Work out the finished part from the listing and answer in its coordinate system (mm). A direction names the side the tool comes from. Round coordinates to 2 decimals unless told otherwise and drop trailing zeros. Write each loop counter-clockwise with the first axis right and the second up, starting at its lowest first coordinate (ties: lowest second). Pieces come first, ordered by that corner, then holes.
1. A tool of negligible diameter and unlimited length cuts with its end or side. For faces 1 (the face through (2.98, -3.03, 3.05)), 2 (the face through (-2, -2, 1.5)), 3 (the face through (-4.25, -0.01, -1.51)), 4 (the face through (-2, -2, 6.5)), from which of +Z, -Z, +X, -X, +Y, -Y can it reach the whole face along a straight path? Write none if from no direction.
2. Find section B-B (x = 0). Write down the section's boundary in (y, z).
3. Straight lines are drawn through the part: probe 1 along X at (y, z) = (-2.25, 3.25); probe 2 along X at (y, z) = (-2, 0.25); probe 3 along Y at (x, z) = (-1.75, 0). For each, find the intervals that lie inside material, in ascending order.
4. Find section A-A (z = 5). Write down the section's boundary in (x, y).
5. Flat-ended cylindrical pins translate along their axes: pin 1 Ø0.5 at (y, z) = (3, 2) entering from -X; pin 2 Ø0.5 at (x, z) = (-3, 0) entering from -Y; pin 3 Ø5 at (y, z) = (0, 2.5) entering from -X; pin 4 Ø1.4 at (y, z) = (-3.5, 1) entering from +X. Find the tip coordinate at first contact, or state that the pin passes through.
6. Determine the mould class of faces 5 (the face through (-0.59, 4.46, -1.51)), 6 (the face through (-1.756, 1.78, 3.965)), 7 (the face through (2, 2, 6.5)) for opening direction X: pulls with the +X half, pulls with the -X half, needs draft (parallel to the pull), parting line crosses it, or undercut.
```python
from build123d import *

# Parameters (mm, degrees)
SKETCH016_R     = 4.5
SKETCH016_R_2   = 2.5
PAD011_DEPTH    = 9
SKETCH018_R     = 5.465451
SKETCH018_R_2   = 4.25
POCKET006_DEPTH = 7
SKETCH019_R     = 4
POCKET007_DEPTH = 4
POCKET008_DEPTH = 9.001
POCKET009_DEPTH = 4


with BuildPart() as part:
    # Sketch016 → Pad011 (new body)
    with BuildSketch(Plane.XY):
        Circle(SKETCH016_R)
        Circle(SKETCH016_R_2, mode=Mode.SUBTRACT)
    extrude(amount=PAD011_DEPTH)

    # Sketch018 (on Face4 of Pad011) → Pocket006 (cut)
    with BuildSketch(Plane.XY.offset(9)):
        Circle(SKETCH018_R)
        Circle(SKETCH018_R_2, mode=Mode.SUBTRACT)
    extrude(amount=-POCKET006_DEPTH, mode=Mode.SUBTRACT)

    # Sketch019 (on Face2 of Pocket006) → Pocket007 (cut)
    with BuildSketch(Plane(origin=(0, 0, 0), x_dir=(1, 0, 0), z_dir=(0, 0, -1))):
        Circle(SKETCH019_R)
    extrude(amount=-POCKET007_DEPTH, mode=Mode.SUBTRACT)

    # Sketch020 (on Face2 of Pocket007) → Pocket008 (cut, through all)
    with BuildSketch(Plane(origin=(0, 0, 0), x_dir=(1, 0, 0), z_dir=(0, 0, -1))):
        with BuildLine():
            ThreePointArc((0.75, 4.1833001327), (0, 4.25), (-0.75, 4.1833001327))
            Line((-0.75, 0.75), (-0.75, 4.1833001327))
            Line((-4.1833001327, 0.75), (-0.75, 0.75))
            ThreePointArc((-4.1833001327, 0.75), (-4.25, 0), (-4.1833001327, -0.75))
            Line((-0.75, -0.75), (-4.1833001327, -0.75))
            Line((-0.75, -4.1833001327), (-0.75, -0.75))
            ThreePointArc((-0.75, -4.1833001327), (0, -4.25), (0.75, -4.1833001327))
            Line((0.75, -0.75), (0.75, -4.1833001327))
            Line((4.1833001327, -0.75), (0.75, -0.75))
            ThreePointArc((4.1833001327, -0.75), (4.25, 0), (4.1833001327, 0.75))
            Line((0.75, 0.75), (4.1833001327, 0.75))
            Line((0.75, 4.1833001327), (0.75, 0.75))
        make_face()
    extrude(amount=-POCKET008_DEPTH, mode=Mode.SUBTRACT)

    # Sketch021 (on Face2 of Pocket008) → Pocket009 (cut)
    with BuildSketch(Plane(origin=(0, 0, 0), x_dir=(0.7071067812, -0.7071067812, 0), z_dir=(0, 0, -1))):
        with BuildLine():
            ThreePointArc((0.75, 4.1833001327), (0, 4.25), (-0.75, 4.1833001327))
            Line((-0.75, 0.75), (-0.75, 4.1833001327))
            Line((-4.1833001327, 0.75), (-0.75, 0.75))
            ThreePointArc((-4.1833001327, 0.75), (-4.25, 0), (-4.1833001327, -0.75))
            Line((-0.75, -0.75), (-4.1833001327, -0.75))
            Line((-0.75, -4.1833001327), (-0.75, -0.75))
            ThreePointArc((-0.75, -4.1833001327), (0, -4.25), (0.75, -4.1833001327))
            Line((0.75, -0.75), (0.75, -4.1833001327))
            Line((4.1833001327, -0.75), (0.75, -0.75))
            ThreePointArc((4.1833001327, -0.75), (4.25, 0), (4.1833001327, 0.75))
            Line((0.75, 0.75), (4.1833001327, 0.75))
            Line((0.75, 4.1833001327), (0.75, 0.75))
        make_face()
    extrude(amount=-POCKET009_DEPTH, mode=Mode.SUBTRACT)


with BuildPart() as part_1:
    # Body006 placement: moved
    add(part.part.moved(Location((0, 0, -2.5))))


solid = part_1.part
```
Worked answers:
1. face 1: +Z, +X, -Y
1. face 2: -Z
1. face 3: +Z, -Z
1. face 4: +Z, +X, -X, +Y, -Y
2. outline: (-4.5, -2.5) - (-4.25, -2.5) - (-4.25, -0.5) - (-4.5, -0.5) - close; (4.25, -2.5) - (4.5, -2.5) - (4.5, -0.5) - (4.25, -0.5) - close
3. probe 1: x = -3.61 to -1.09, 1.09 to 3.61
3. probe 2: x = -3.75 to -3.46, 3.46 to 3.75
3. probe 3: y = -3.87 to -3.6, 3.6 to 3.87
4. outline: (-4.18, -0.75) arc R4.25 ccw to (-0.75, -4.18) - (-0.75, -2.38) arc R2.5 cw to (-2.38, -0.75) - close; (-4.18, 0.75) - (-2.38, 0.75) arc R2.5 cw to (-0.75, 2.38) - (-0.75, 4.18) arc R4.25 ccw to start; (0.75, -4.18) arc R4.25 ccw to (4.18, -0.75) - (2.38, -0.75) arc R2.5 cw to (0.75, -2.38) - close; (0.75, 2.38) arc R2.5 cw to (2.38, 0.75) - (4.18, 0.75) arc R4.25 ccw to (0.75, 4.18) - close
5. pin 1: stops at x = -3.24
5. pin 2: passes through
5. pin 3: stops at x = -4.18
5. pin 4: stops at x = 3
6. face 5: parting line crosses it
6. face 6: undercut
6. face 7: needs draft
